from build123d import *

# Parameters (mm, degrees)
SKETCH_1_W               = 1225
SKETCH_1_H               = 370
EXTRUDE_1_DEPTH          = 16
SKETCH_2_W               = 280
SKETCH_2_H               = 280
EXTRUDE_2_DEPTH          = 10
SKETCH_3_R               = 85
SKETCH_3_R_2             = 75
EXTRUDE_3_DEPTH          = 135
EXTRUDE_4_DEPTH          = 135
PATTERN_CIRCULAR_1_COUNT = 8
SKETCH_5_W               = 280
SKETCH_5_H               = 280
SKETCH_5_R               = 56
EXTRUDE_5_DEPTH          = 35
SKETCH_6_R               = 105
CUT_EXTRUDE_1_DEPTH      = 8
SKETCH_7_W               = 16
SKETCH_7_H               = 1195
EXTRUDE_8_DEPTH          = 180
EXTRUDE_START            = 16
SKETCH_8_W               = 370
SKETCH_8_H               = 1175
SKETCH_8_R               = 105
EXTRUDE_9_DEPTH          = 16
EXTRUDE_START_2          = 5
SKETCH_9_W               = 360
SKETCH_9_H               = 280
SKETCH_9_R               = 105
EXTRUDE_10_DEPTH         = 5


with BuildPart() as part:
    # 草图1 → 凸台-拉伸1 (new body)
    with BuildSketch(Plane(origin=(0, 0, 0), x_dir=(0, 0, -1), z_dir=(0, 1, 0))):
        Rectangle(SKETCH_1_W, SKETCH_1_H)
    extrude(amount=EXTRUDE_1_DEPTH)

    # 草图2 → 凸台-拉伸2 (add)
    with BuildSketch(Plane(origin=(0, 16, 0), x_dir=(1, 0, 0), z_dir=(0, 1, 0))):
        Rectangle(SKETCH_2_W, SKETCH_2_H)
    extrude(amount=EXTRUDE_2_DEPTH)

    # 草图3 → 凸台-拉伸3 (add)
    with BuildSketch(Plane(origin=(0, 26, 0), x_dir=(1, 0, 0), z_dir=(0, 1, 0))):
        with Locations(Location((0, 0, 0), (0, 0, 270))):
            Circle(SKETCH_3_R)
        with Locations(Location((0, 0, 0), (0, 0, 270))):
            Circle(SKETCH_3_R_2, mode=Mode.SUBTRACT)
    extrude(amount=EXTRUDE_3_DEPTH)

    # 草图4 → 凸台-拉伸4 (add)
    with BuildSketch(Plane(origin=(0, 26, 0), x_dir=(1, 0, 0), z_dir=(0, 1, 0))):
        with BuildLine():
            Line((27.852368346, 80.307195054), (52.577523517, 139.999))
            Line((52.577523517, 139.999), (61.816318842, 136.172165676))
            Line((61.816318842, 136.172165676), (37.091163671, 76.480360731))
            ThreePointArc((37.091163671, 76.480360731), (32.528091751, 78.529760263), (27.852368346, 80.307195054))
        make_face()
    extrude_4 = extrude(amount=EXTRUDE_4_DEPTH)

    # 阵列(圆周)1: 凸台-拉伸4 ×8 about axis
    pattern_circular_1_axis = Axis((0, 0, 0), (0, 1, 0))
    for i in range(1, PATTERN_CIRCULAR_1_COUNT):
        add(extrude_4.rotate(pattern_circular_1_axis, i * 360 / PATTERN_CIRCULAR_1_COUNT))

    # 草图5 → 凸台-拉伸5 (add)
    with BuildSketch(Plane(origin=(0, 161, 0), x_dir=(1, 0, 0), z_dir=(0, 1, 0))):
        Rectangle(SKETCH_5_W, SKETCH_5_H)
        with Locations(Location((0, 0, 0), (0, 0, 270))):
            Circle(SKETCH_5_R, mode=Mode.SUBTRACT)
    extrude(amount=EXTRUDE_5_DEPTH)

    # 草图6 → 切除-拉伸1 (cut)
    with BuildSketch(Plane(origin=(0, 196, 0), x_dir=(1, 0, 0), z_dir=(0, 1, 0))):
        with Locations(Location((0, 0, 0), (0, 0, 270))):
            Circle(SKETCH_6_R)
    extrude(amount=-CUT_EXTRUDE_1_DEPTH, mode=Mode.SUBTRACT)

    # 草图7 → 凸台-拉伸8 (add)
    with BuildSketch(Plane(origin=(0, 16, 0), x_dir=(1, 0, 0), z_dir=(0, 1, 0))):
        with Locations((-148, 0)):
            Rectangle(SKETCH_7_W, SKETCH_7_H)
        with Locations((148, 0)):
            Rectangle(SKETCH_7_W, SKETCH_7_H)
    extrude(amount=EXTRUDE_8_DEPTH)

    # 草图8 → 凸台-拉伸9 (add)
    with BuildSketch(Plane(origin=(0, 196, 0), x_dir=(1, 0, 0), z_dir=(0, 1, 0)).offset(EXTRUDE_START)):
        Rectangle(SKETCH_8_W, SKETCH_8_H)
        with Locations(Location((0, 0, 0), (0, 0, 270))):
            Circle(SKETCH_8_R, mode=Mode.SUBTRACT)
    extrude(amount=-EXTRUDE_9_DEPTH)

    # 草图9 → 凸台-拉伸10 (add)
    with BuildSketch(Plane(origin=(0, 212, 0), x_dir=(1, 0, 0), z_dir=(0, 1, 0)).offset(EXTRUDE_START_2)):
        Rectangle(SKETCH_9_W, SKETCH_9_H)
        with Locations(Location((0, 0, 0), (0, 0, 270))):
            Circle(SKETCH_9_R, mode=Mode.SUBTRACT)
    extrude(amount=-EXTRUDE_10_DEPTH)


solid = part.part
Geometry check sheet. Reference: the model listing, model coordinates, mm. A direction names the side the tool comes from. Round coordinates to 2 decimals unless told otherwise and drop trailing zeros. Write each loop counter-clockwise with the first axis right and the second up, starting at its lowest first coordinate (ties: lowest second). Pieces come first, ordered by that corner, then holes. Notation, with made-up numbers: (-37, 1.25) -> (17, 1.25) arc R27 ccw to (17, 32.25) -> close; hole circle Ø6 at (35, 32.5). An arc over 180 degrees is marked (long way). One line per item, written item: value. Start each with the question number.
(1) Cross-section at A-A, the plane z = 408. Record the cut outline in (x, y), and give its area (3 significant figures).
(2) Access from +Z, -Z, +X, -X, +Y, -Y to the whole of each face (thin tool, end or side, straight path). Record for faces 4 (the flat face through (-3, 16, 145)), 5 (the flat face through (-105.91, 92.56, 49.28)), 6 (the flat face through (-156, 105, 8)), 7 (the flat face through (105.91, 92.56, -49.28)), 8 (the flat face through (-3, 0, 9)).
(3) Draft check along Y on faces 1 (the flat face through (-2, 178, 140)), 2 (the cylindrical face through (31.54, 202.7, 100.15)), 3 (the flat face through (-45, 188, 45)). Enter one of: +Y half, -Y half, draft (parallel to the pull), parting line (faces both ways), or undercut.
(4) Cross-section at D-D, the plane y = 51.5. Give the number of separate pieces and of enclosed holes in the cut face, and give its area (3 significant figures).
(5) Cross-section at C-C, the plane x = -119.5. Record the cut outline in (y, z), and give its area (3 significant figures).
(6) Scan lines: line 1 (X direction, y = 125, z = 0); line 2 (Z direction, x = -0.5, y = 103); line 3 (Y direction, x = 26, z = -334.5). Record each from-to range of solid material in increasing order. Write a range as [from, to].
(7) Go/stop test with flat-tipped pins: pin 1 Ø5 at (x, y) = (-146, 123.5) entering from +Z; pin 2 Ø17.5 at (x, y) = (-25, 202) entering from -Z; pin 3 Ø8 at (x, y) = (-59, 20.5) entering from -Z; pin 4 Ø1.5 at (x, z) = (1, -355) entering from -Y. Record where each tip stops, or that it passes through.
(8) Cross-section at B-B, the plane y = 177.5. Record the cut outline in (x, z).
Answer:
1. outline: (-185, 0) -> (185, 0) -> (185, 16) -> (156, 16) -> (156, 196) -> (185, 196) -> (185, 212) -> (-185, 212) -> (-185, 196) -> (-156, 196) -> (-156, 16) -> (-185, 16) -> close; hole (-140, 16) -> (140, 16) -> (140, 196) -> (-140, 196) -> close
1. area: 17,600 mm²
2. face 4: none
2. face 5: +Z
2. face 6: +Z, -Z, -X
2. face 7: -Z
2. face 8: +Z, -Z, +X, -X, -Y
3. face 1: undercut
3. face 2: draft
3. face 3: +Y half
4. separate pieces: 3
4. enclosed holes: 1
4. area: 48,400 mm²
5. outline: (0, -612.5) -> (16, -612.5) -> (16, -140) -> (26, -140) -> (26, -54.91) -> (161, -54.91) -> (161, -140) -> (196, -140) -> (196, -587.5) -> (212, -587.5) -> (212, -140) -> (217, -140) -> (217, 140) -> (212, 140) -> (212, 587.5) -> (196, 587.5) -> (196, 140) -> (161, 140) -> (161, 54.91) -> (26, 54.91) -> (26, 140) -> (16, 140) -> (16, 612.5) -> (0, 612.5) -> close; hole (26, -44.09) -> (161, -44.09) -> (161, 44.09) -> (26, 44.09) -> close
5. area: 55,300 mm²
6. line 1: [-156, -140], [-85, -75], [75, 85], [140, 156]
6. line 2: [-85, -75], [75, 85]
6. line 3: [0, 16], [196, 212]
7. pin 1: z = 597.5
7. pin 2: z = -587.5
7. pin 3: z = -140
7. pin 4: y = 0
8. outline: (-156, -597.5) -> (-140, -597.5) -> (-140, -140) -> (140, -140) -> (140, -597.5) -> (156, -597.5) -> (156, 597.5) -> (140, 597.5) -> (140, 140) -> (-140, 140) -> (-140, 597.5) -> (-156, 597.5) -> close; hole circle Ø112 at (0, 0)
